Can you work these out from the model? Positions are in its coordinate system, mm. Face numbers are marked on the shaded views. Coordinates: 2 decimals unless noted, no trailing zeros. Write each loop counter-clockwise with the first axis right and the second up, starting at its lowest first coordinate (ties: lowest second). Pieces come first, ordered by that corner, then holes. Notation, with made-up numbers: M 33,74.5 L 44,74.5 A22 cw 44,100.5 Z; hole C 53,-5.75 d5. An arc over 180 degrees is marked long. Use one line per item in the form item = value. Start each with the question number.
```python
from build123d import *

# Parameters (mm, degrees)
BOSS_EXTRUDE1_DEPTH = 8
SKETCH3_W           = 7
SKETCH3_H           = 0.75
BOSS_EXTRUDE2_DEPTH = 8
BOSS_EXTRUDE3_DEPTH = 8
CUT_EXTRUDE1_REACH  = 21.747
SKETCH2_R           = 1.55


with BuildPart() as part:
    # Sketch1 → Boss-Extrude1 (new body)
    with BuildSketch(Plane(origin=(0, 0, 0), x_dir=(1, 0, 0), z_dir=(0, 1, 0))):
        with BuildLine():
            Line((-0.73791447, 0.195), (-1.26208553, 0.195))
            ThreePointArc((-1.26208553, 0.195), (-1.368151547, 0.151066017), (-1.41208553, 0.045))
            ThreePointArc((-1.41208553, 0.045), (-1.459490829, -0.139768303), (-1.541118048, -0.312173597))
            ThreePointArc((-1.541118048, -0.312173597), (-1.740415087, -0.490551397), (-2, -0.555))
            Line((-2, -0.555), (-2, -5.555))
            Line((-2, -5.555), (14, -5.555))
            Line((14, -5.555), (14, -0.555))
            ThreePointArc((14, -0.555), (13.740415087, -0.490551397), (13.541118048, -0.312173597))
            ThreePointArc((13.541118048, -0.312173597), (13.459490829, -0.139768303), (13.41208553, 0.045))
            ThreePointArc((13.41208553, 0.045), (13.368151547, 0.151066017), (13.26208553, 0.195))
            Line((13.26208553, 0.195), (12.73791447, 0.195))
            ThreePointArc((12.73791447, 0.195), (12.631848453, 0.151066017), (12.58791447, 0.045))
            ThreePointArc((12.58791447, 0.045), (12.540509171, -0.139768303), (12.458881952, -0.312173597))
            ThreePointArc((12.458881952, -0.312173597), (12.259584913, -0.490551397), (12, -0.555))
            ThreePointArc((12, -0.555), (11.740415087, -0.490551397), (11.541118048, -0.312173597))
            ThreePointArc((11.541118048, -0.312173597), (11.459490829, -0.139768303), (11.41208553, 0.045))
            ThreePointArc((11.41208553, 0.045), (11.368151547, 0.151066017), (11.26208553, 0.195))
            Line((11.26208553, 0.195), (10.73791447, 0.195))
            ThreePointArc((10.73791447, 0.195), (10.631848453, 0.151066017), (10.58791447, 0.045))
            ThreePointArc((10.58791447, 0.045), (10.540509171, -0.139768303), (10.458881952, -0.312173597))
            ThreePointArc((10.458881952, -0.312173597), (10.259584913, -0.490551397), (10, -0.555))
            ThreePointArc((10, -0.555), (9.740415087, -0.490551397), (9.541118048, -0.312173597))
            ThreePointArc((9.541118048, -0.312173597), (9.459490829, -0.139768303), (9.41208553, 0.045))
            ThreePointArc((9.41208553, 0.045), (9.368151547, 0.151066017), (9.26208553, 0.195))
            Line((9.26208553, 0.195), (8.73791447, 0.195))
            ThreePointArc((8.73791447, 0.195), (8.631848453, 0.151066017), (8.58791447, 0.045))
            ThreePointArc((8.58791447, 0.045), (8.540509171, -0.139768303), (8.458881952, -0.312173597))
            ThreePointArc((8.458881952, -0.312173597), (8.259584913, -0.490551397), (8, -0.555))
            ThreePointArc((8, -0.555), (7.740415087, -0.490551397), (7.541118048, -0.312173597))
            ThreePointArc((7.541118048, -0.312173597), (7.459490829, -0.139768303), (7.41208553, 0.045))
            ThreePointArc((7.41208553, 0.045), (7.368151547, 0.151066017), (7.26208553, 0.195))
            Line((7.26208553, 0.195), (6.73791447, 0.195))
            ThreePointArc((6.73791447, 0.195), (6.631848453, 0.151066017), (6.58791447, 0.045))
            ThreePointArc((6.58791447, 0.045), (6.540509171, -0.139768303), (6.458881952, -0.312173597))
            ThreePointArc((6.458881952, -0.312173597), (6.259584913, -0.490551397), (6, -0.555))
            ThreePointArc((6, -0.555), (5.740415087, -0.490551397), (5.541118048, -0.312173597))
            ThreePointArc((5.541118048, -0.312173597), (5.459490829, -0.139768303), (5.41208553, 0.045))
            ThreePointArc((5.41208553, 0.045), (5.368151547, 0.151066017), (5.26208553, 0.195))
            Line((5.26208553, 0.195), (4.73791447, 0.195))
            ThreePointArc((4.73791447, 0.195), (4.631848453, 0.151066017), (4.58791447, 0.045))
            ThreePointArc((4.58791447, 0.045), (4.540509171, -0.139768303), (4.458881952, -0.312173597))
            ThreePointArc((4.458881952, -0.312173597), (4.259584913, -0.490551397), (4, -0.555))
            ThreePointArc((4, -0.555), (3.740415087, -0.490551397), (3.541118048, -0.312173597))
            ThreePointArc((3.541118048, -0.312173597), (3.459490829, -0.139768303), (3.41208553, 0.045))
            ThreePointArc((3.41208553, 0.045), (3.368151547, 0.151066017), (3.26208553, 0.195))
            Line((3.26208553, 0.195), (2.73791447, 0.195))
            ThreePointArc((2.73791447, 0.195), (2.631848453, 0.151066017), (2.58791447, 0.045))
            ThreePointArc((2.58791447, 0.045), (2.540509171, -0.139768303), (2.458881952, -0.312173597))
            ThreePointArc((2.458881952, -0.312173597), (2.259584913, -0.490551397), (2, -0.555))
            ThreePointArc((2, -0.555), (1.740415087, -0.490551397), (1.541118048, -0.312173597))
            ThreePointArc((1.541118048, -0.312173597), (1.459490829, -0.139768303), (1.41208553, 0.045))
            ThreePointArc((1.41208553, 0.045), (1.368151547, 0.151066017), (1.26208553, 0.195))
            Line((1.26208553, 0.195), (0.73791447, 0.195))
            ThreePointArc((0.73791447, 0.195), (0.631848453, 0.151066017), (0.58791447, 0.045))
            ThreePointArc((0.58791447, 0.045), (0.540509171, -0.139768303), (0.458881952, -0.312173597))
            ThreePointArc((0.458881952, -0.312173597), (0.259584913, -0.490551397), (0, -0.555))
            ThreePointArc((0, -0.555), (-0.259584913, -0.490551397), (-0.458881952, -0.312173597))
            ThreePointArc((-0.458881952, -0.312173597), (-0.540509171, -0.139768303), (-0.58791447, 0.045))
            ThreePointArc((-0.58791447, 0.045), (-0.631848453, 0.151066017), (-0.73791447, 0.195))
        make_face()
    extrude(amount=BOSS_EXTRUDE1_DEPTH)

    # Sketch3 → Boss-Extrude2 (add)
    with BuildSketch(Plane(origin=(0, 8, 0), x_dir=(1, 0, 0), z_dir=(0, 1, 0))):
        with Locations((10.5, -0.18)):
            Rectangle(SKETCH3_W, SKETCH3_H)
    extrude(amount=-BOSS_EXTRUDE2_DEPTH)

    # Sketch4 → Boss-Extrude3 (add)
    with BuildSketch(Plane(origin=(0, 8, 0), x_dir=(1, 0, 0), z_dir=(0, 1, 0))):
        Polygon((6.73791447, 0.195), (6.73791447, 0.845), (-2, 0.845), (-2, 5.845), (14, 5.845), (14, 0.195), align=None)
    extrude(amount=-BOSS_EXTRUDE3_DEPTH)

    # Sketch2 → Cut-Extrude1 (cut, up to next)
    with BuildSketch(Plane.XY.offset(5.555), mode=Mode.PRIVATE) as cut_extrude1_sk1:
        with Locations((10, 4)):
            Circle(SKETCH2_R)
    cut_extrude1_tool1 = extrude(cut_extrude1_sk1.sketch, amount=-CUT_EXTRUDE1_REACH, mode=Mode.PRIVATE) & part.part
    add(cut_extrude1_tool1.solids().sort_by_distance((10, 4, 5.555))[0], mode=Mode.SUBTRACT)


solid = part.part
```
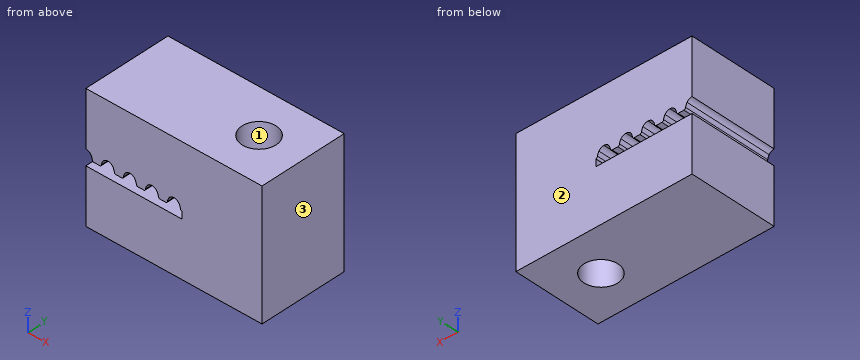
1) Please list where these lines run through material, in increasing order: line 1 (Y direction, x = 10, z = 2.5); line 2 (Z direction, x = 6, y = 2.75) (3 decimals); line 3 (Z direction, x = 1, y = 5) (3 decimals).
2) Suppose I cut it at A-A on x = 10. Please give me the cut outline in (y, z) (3 decimals), and give its area (3 significant figures).
3) Will this pin go through, and if not, where does the flat tip stop? pin 1 Ø1 at (x, y) = (9, 4) entering from -Z.
4) If we mould it in two halves opening along X, with no side actions, what happens to the marked faces 1, 2 and 3? For each: +X half, -X half, draft (parallel to the pull), parting line (faces both ways), or undercut.
5) Suppose I cut it at B-B on z = 4.75. Please give me the cut outline in (x, y), and give its area (3 significant figures).
Computed values:
q1.line_1 = 0 to 2.45, 5.55 to 8
q1.line_2 = -5.845 to -0.845, 0.555 to 5.555
q1.line_3 = -5.845 to -0.845, -0.195 to 5.555
q2.outline = M 0,-5.845 L 2.45,-5.845 L 2.45,5.555 L 0,5.555 Z; M 5.55,-5.845 L 8,-5.845 L 8,5.555 L 5.55,5.555 Z
q2.area = 55.9 mm²
q3.pin_1 = through
q4.face_1 = undercut
q4.face_2 = draft
q4.face_3 = +X half
q5.outline = M -2,0 L 14,0 L 14,8 L -2,8 Z; hole C 10,4 d3.1
q5.area = 120 mm²
